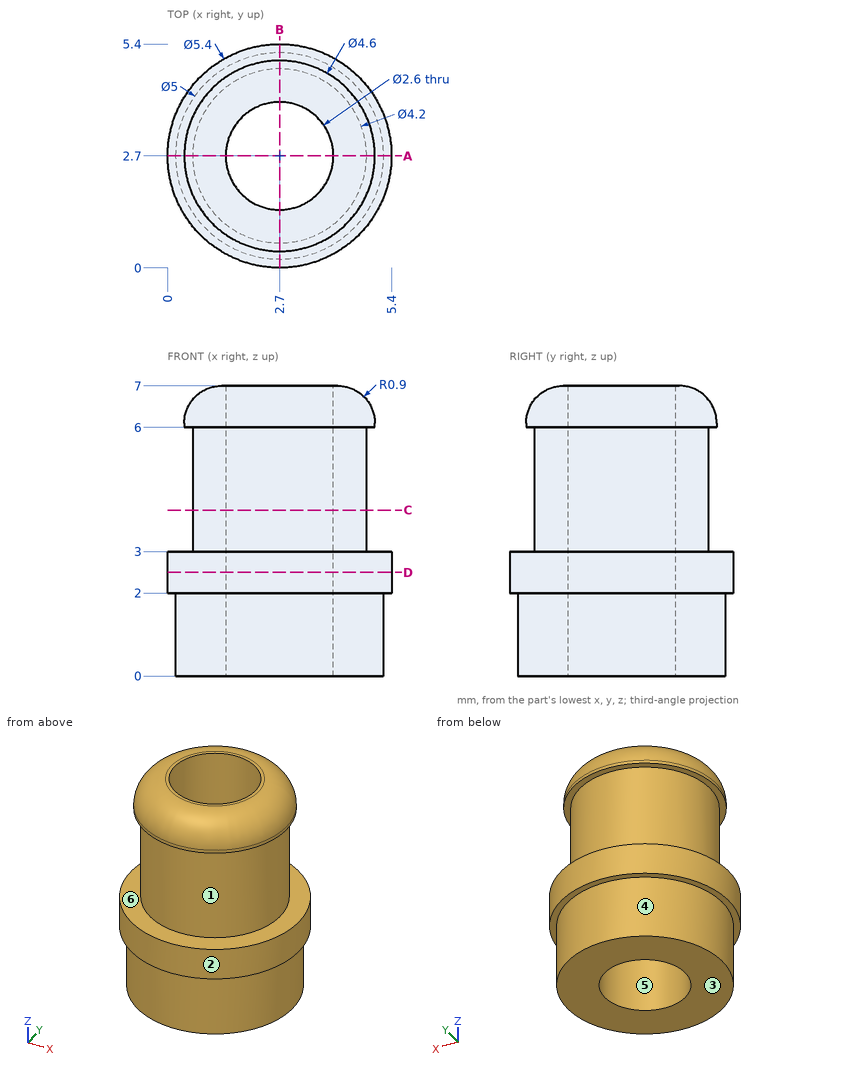
Job drawing, mm, ordinate dimensions from the low corner. One solid piece. A direction names the side the tool comes from. Round coordinates to 2 decimals unless told otherwise and drop trailing zeros. Write each loop counter-clockwise with the first axis right and the second up, starting at its lowest first coordinate (ties: lowest second). Pieces come first, ordered by that corner, then holes. Notation, with made-up numbers: M -29,40 L 11,40 A20 ccw 11,46 Z; hole C 16,37.5 d9. An arc over 180 degrees is marked long. Return JSON: item names as keys, results as strings. Group by question number.
(1) Saw through at C-C on z = 4. Write the cut outline in (x, y).
(2) Which spindle directions (+Z, -Z, +X, -X, +Y, -Y) get a long thin tool onto all of the face, cutting with end or side? Do the marked faces 4, 5 and 6. Say none if no direction does.
(3) Saw through at D-D on z = 2.5. Write the cut outline in (x, y).
(4) Two-plate mould, pull along Z, no slides. Class the marked faces 1, 2 and 3: +Z half, -Z half, draft (parallel to the pull), parting line (faces both ways), or undercut.
(5) Saw through at A-A on y = 2.7. Write the cut outline in (x, z), then the cut area to 3 significant figures.
(6) Drill centre lines: probe 1 along Y at (x, z) = (2.7, 5.5); probe 2 along Y at (x, z) = (2.7, 2.25); probe 3 along Z at (x, y) = (4.4, 0.75). Where is each one in solid material? Low to high.
(7) Pin check, flat tips, straight feed: pin 1 Ø2 at (x, z) = (1.5, 3.5) entering from +Y; pin 2 Ø2 at (x, z) = (1.5, 5.5) entering from -Y; pin 3 Ø1.5 at (x, z) = (4, 2.5) entering from -Y. Stop position of each tip, or through.
Returned:
{
 "1": {"outline": "C 2.7,2.7 d4.2; hole C 2.7,2.7 d2.6"},
 "2": {"face 4": "-Z", "face 5": "+Z, -Z", "face 6": "none"},
 "3": {"outline": "C 2.7,2.7 d5.4; hole C 2.7,2.7 d2.6"},
 "4": {"face 1": "undercut", "face 2": "draft", "face 3": "-Z half"},
 "5": {"outline": "M 0,2 L 0.2,2 L 0.2,0 L 1.4,0 L 1.4,7 L 1.3,7 A0.9 ccw 0.4,6.1 L 0.4,6 L 0.6,6 L 0.6,3 L 0,3 Z; M 4,0 L 5.2,0 L 5.2,2 L 5.4,2 L 5.4,3 L 4.8,3 L 4.8,6 L 5,6 L 5,6.1 A0.9 ccw 4.1,7 L 4,7 Z", "area": "14.1 mm²"},
 "6": {"probe 1": "0.6 to 1.4, 4 to 4.8", "probe 2": "0 to 1.4, 4 to 5.4", "probe 3": "2 to 3"},
 "7": {"pin 1": "y = 5.38", "pin 2": "y = 0.42", "pin 3": "y = 0.06"}
}
